Here's how the part is built. I have some questions about the finished solid (model axes, mm). A direction names the side the tool comes from. Coordinates: 2 decimals unless noted, no trailing zeros. Write each loop counter-clockwise with the first axis right and the second up, starting at its lowest first coordinate (ties: lowest second). Pieces come first, ordered by that corner, then holes.
from build123d import *

# Parameters (mm, degrees)
SKETCH_1_R      = 20
SKETCH_1_R_2    = 2
SKETCH_1_R_3    = 4
EXTRUDE_1_DEPTH = 10
SKETCH_2_R      = 22.5
SKETCH_2_R_2    = 4
SKETCH_2_R_3    = 2
EXTRUDE_2_DEPTH = 1
EXTRUDE_START   = 1
SKETCH_3_R      = 22.5
SKETCH_3_R_2    = 4
SKETCH_3_R_3    = 2
EXTRUDE_3_DEPTH = 1


with BuildPart() as part:
    # 草图1 → 凸台-拉伸1 (new body)
    with BuildSketch(Plane(origin=(0, 0, 0), x_dir=(1, 0, 0), z_dir=(0, 1, 0))):
        with Locations(Location((0, 0, 0), (0, 0, 270))):
            Circle(SKETCH_1_R)
        with Locations(Location((0, 15, 0), (0, 0, 270))):
            Circle(SKETCH_1_R_2, mode=Mode.SUBTRACT)
        with Locations(Location((15, 0, 0), (0, 0, 270))):
            Circle(SKETCH_1_R_2, mode=Mode.SUBTRACT)
        with Locations(Location((0, -15, 0), (0, 0, 270))):
            Circle(SKETCH_1_R_2, mode=Mode.SUBTRACT)
        with Locations(Location((-15, 0, 0), (0, 0, 270))):
            Circle(SKETCH_1_R_2, mode=Mode.SUBTRACT)
        with Locations(Location((0, 0, 0), (0, 0, 270))):
            Circle(SKETCH_1_R_3, mode=Mode.SUBTRACT)
    extrude(amount=EXTRUDE_1_DEPTH)

    # 草图2 → 凸台-拉伸2 (add)
    with BuildSketch(Plane(origin=(0, 10, 0), x_dir=(1, 0, 0), z_dir=(0, 1, 0))):
        with Locations(Location((0, 0, 0), (0, 0, 270))):
            Circle(SKETCH_2_R)
        with Locations(Location((0, 0, 0), (0, 0, 270))):
            Circle(SKETCH_2_R_2, mode=Mode.SUBTRACT)
        with Locations(Location((-15, 0, 0), (0, 0, 270))):
            Circle(SKETCH_2_R_3, mode=Mode.SUBTRACT)
        with Locations(Location((0, 15, 0), (0, 0, 270))):
            Circle(SKETCH_2_R_3, mode=Mode.SUBTRACT)
        with Locations(Location((15, 0, 0), (0, 0, 270))):
            Circle(SKETCH_2_R_3, mode=Mode.SUBTRACT)
        with Locations(Location((0, -15, 0), (0, 0, 270))):
            Circle(SKETCH_2_R_3, mode=Mode.SUBTRACT)
    extrude(amount=EXTRUDE_2_DEPTH)

    # 草图3 → 凸台-拉伸3 (add)
    with BuildSketch(Plane.XZ.offset(EXTRUDE_START)):
        with Locations(Location((0, 0, 0), (0, 0, 90))):
            Circle(SKETCH_3_R)
        with Locations(Location((0, 0, 0), (0, 0, 270))):
            Circle(SKETCH_3_R_2, mode=Mode.SUBTRACT)
        with Locations(Location((15, 0, 0), (0, 0, 270))):
            Circle(SKETCH_3_R_3, mode=Mode.SUBTRACT)
        with Locations(Location((0, -15, 0), (0, 0, 270))):
            Circle(SKETCH_3_R_3, mode=Mode.SUBTRACT)
        with Locations(Location((-15, 0, 0), (0, 0, 270))):
            Circle(SKETCH_3_R_3, mode=Mode.SUBTRACT)
        with Locations(Location((0, 15, 0), (0, 0, 270))):
            Circle(SKETCH_3_R_3, mode=Mode.SUBTRACT)
    extrude(amount=-EXTRUDE_3_DEPTH)


solid = part.part
1. I want a section at B-B (z = 0). List the corners of the cut face in (x, y) for me.
2. For pin 1 Ø1 at (x, y) = (3, 7.5) entering from +Z; pin 2 Ø1 at (y, z) = (8, 6) entering from -X; pin 3 Ø1 at (x, y) = (10.5, 4.5) entering from +Z, each with a flat end and sliding along its axis, tell me the tip position at first contact or that it passes through.
3. Thinking about a two-plate mould opening in Y: for faces 3 (the face through (-1.6, 10, -20.1)), 4 (the face through (-8.618, 10.493, 20.784)), 5 (the face through (5, -1, 0)), 6 (the face through (1.6, 0, -20.1)), which applies, pulls with the +Y half, pulls with the -Y half, needs draft (parallel to the pull), parting line crosses it, or undercut?
4. I want a section at D-D (x = -15). List the corners of the cut face in (y, z) for me, then the cut area to 3 significant figures.
5. On a 3-axis mill with a long thin cutter (end or side, diameter ignored), from which of +Z, -Z, +X, -X, +Y, -Y can I reach the whole of each face in a straight line? I mean faces 1 (the face through (8.618, -0.507, 20.784)), 2 (the face through (-19.524, 4.93, -4.336)). Say none if no direction works.
6. If I drill on line 1 (X direction, y = -0.5, z = 0); line 2 (X direction, y = 7, z = 0); line 3 (Y direction, x = -13, z = 18), over which ranges is the centre line in solid material (lowest first)?
7. I want a section at C-C (z = 15). List the corners of the cut face in (x, y) for me.
Response values:
1. outline: (-22.5, -1) - (-17, -1) - (-17, 11) - (-22.5, 11) - (-22.5, 10) - (-20, 10) - (-20, 0) - (-22.5, 0) - close; (-13, -1) - (-4, -1) - (-4, 11) - (-13, 11) - close; (4, -1) - (13, -1) - (13, 11) - (4, 11) - close; (17, -1) - (22.5, -1) - (22.5, 0) - (20, 0) - (20, 10) - (22.5, 10) - (22.5, 11) - (17, 11) - close
2. pin 1: stops at z = 19.84
2. pin 2: stops at x = -19.23
2. pin 3: stops at z = 17.32
3. face 3: undercut
3. face 4: needs draft
3. face 5: pulls with the -Y half
3. face 6: undercut
4. outline: (-1, -16.77) - (0, -16.77) - (0, -13.23) - (10, -13.23) - (10, -16.77) - (11, -16.77) - (11, -2) - (-1, -2) - close; (-1, 2) - (11, 2) - (11, 16.77) - (10, 16.77) - (10, 13.23) - (0, 13.23) - (0, 16.77) - (-1, 16.77) - close
4. area: 284 mm2
5. face 1: +Y, -Y
5. face 2: none
6. line 1: x = -22.5 to -17, -13 to -4, 4 to 13, 17 to 22.5
6. line 2: x = -20 to -17, -13 to -4, 4 to 13, 17 to 20
6. line 3: y = -1 to 0, 10 to 11
7. outline: (-16.77, -1) - (-2, -1) - (-2, 11) - (-16.77, 11) - (-16.77, 10) - (-13.23, 10) - (-13.23, 0) - (-16.77, 0) - close; (2, -1) - (16.77, -1) - (16.77, 0) - (13.23, 0) - (13.23, 10) - (16.77, 10) - (16.77, 11) - (2, 11) - close
